Geometry: final body of the model. Coordinates: model frame, mm. A direction names the side the tool comes from. Give positions to 0.01 mm unless a question says otherwise; leave off trailing zeros. Order: outer loops, then holes, each group sorted by start corner. A loop starts at its lowest first (then second) coordinate and runs counter-clockwise, first axis right, second up. Notation, with made-up numbers: M 75.25,24.25 L 89.25,24.25 A9 cw 89.25,30.25 Z; hole C 31.5,70.25 d3. An arc over 180 degrees is marked long. Use CSV: the item, a comma, the result in double quotes.
```python
from build123d import *

# Parameters (mm, degrees)
F0_W     = 76.2
F0_H     = 101.6
F1_DEPTH = 10.16
F2_W     = 5.08
F2_H     = 5.08
F3_DEPTH = 50.8
F4_R     = 5.08


with BuildPart() as f1:
    # F0 (on Top) → F1 (new body)
    with BuildSketch(Plane.XY):
        Rectangle(F0_W, F0_H)
    extrude(amount=F1_DEPTH)

    # F2 (on face) → F3 (join)
    with BuildSketch(Plane.XY.offset(10.16)):
        with Locations((35.56, 48.26)):
            Rectangle(F2_W, F2_H)
        with Locations((35.56, -48.26)):
            Rectangle(F2_W, F2_H)
        with Locations((-35.56, 48.26)):
            Rectangle(F2_W, F2_H)
        with Locations((-35.56, -48.26)):
            Rectangle(F2_W, F2_H)
    extrude(amount=F3_DEPTH)

    # F4
    f4_edges = [f1.edges().sort_by_distance(p)[0] for p in [
        (0, 50.8, 0),
        (38.1, 0, 0),
        (0, -50.8, 0),
        (-38.1, 0, 0),
    ]]
    fillet(f4_edges, radius=F4_R)


solid = f1.part
```
1. Section B-B, the plane y = -3.5. Return the cut outline in (x, z).
Answer:
outline,"M -38.1,5.08 A5.08 ccw -33.02,0 L 33.02,0 A5.08 ccw 38.1,5.08 L 38.1,10.16 L -38.1,10.16 Z"
2. Reachability of faces 4 (the face through (-36.651, 0.711, 1.528)), 5 (the face through (33.02, 48, 35)), 6 (the face through (36, 45.72, 35)) from +Z, -Z, +X, -X, +Y, -Y: full face, straight path, thin tool, end or side. Return the list, or none.
Answer:
face 4,"-Z, -X, +Y, -Y"
face 5,"+Z, +Y, -Y"
face 6,"+Z, +X, -X"
3. Pull-direction query (Y, two-part tool) for faces 1 (the face through (0.533, -49.351, 1.528)), 2 (the face through (0, 1, 0)), 3 (the face through (-36, 45.72, 35)); classes: +Y half, -Y half, draft (parallel to the pull), parting line (faces both ways), or undercut.
Answer:
face 1,"-Y half"
face 2,"draft"
face 3,"undercut"
4. Section A-A, the plane z = 52.5. Return the cut outline in (x, y), plus the area to 3 significant figures.
Answer:
outline,"M -38.1,-50.8 L -33.02,-50.8 L -33.02,-45.72 L -38.1,-45.72 Z; M -38.1,45.72 L -33.02,45.72 L -33.02,50.8 L -38.1,50.8 Z; M 33.02,-50.8 L 38.1,-50.8 L 38.1,-45.72 L 33.02,-45.72 Z; M 33.02,45.72 L 38.1,45.72 L 38.1,50.8 L 33.02,50.8 Z"
area,"103 mm2"
5. Line query: line 1 (Y direction, x = 34.5, z = 20.5); line 2 (Z direction, x = -29.5, y = 27); line 3 (Z direction, x = 35, y = 25.5). Output: solid intervals per line, ascending.
Answer:
line 1,"-50.8 to -45.72, 45.72 to 50.8"
line 2,"0 to 10.16"
line 3,"0.4 to 10.16"
6. Section C-C, the plane x = 28.5. Return the cut outline in (y, z).
Answer:
outline,"M -50.8,5.08 A5.08 ccw -45.72,0 L 45.72,0 A5.08 ccw 50.8,5.08 L 50.8,10.16 L -50.8,10.16 Z"
